Can you work these out from the model? Positions are in its coordinate system, mm. A direction names the side the tool comes from. Round coordinates to 2 decimals unless told otherwise and drop trailing zeros. Order: outer loops, then holes, each group sorted by start corner. A loop starts at its lowest first (then second) coordinate and runs counter-clockwise, first axis right, second up. Notation, with made-up numbers: (33.5, -12) - (48.5, -12) arc R27 cw to (48.5, 16) - close; hole circle Ø10 at (-23, -36). An arc over 180 degrees is marked (long way). Write item = value, one per line.
Autodesk Inventor part; units mm, degrees
ref_plane "Work Plane1" through (0, 0, 10) normal (0, 0, 1) x (1, 0, 0)
ref_plane "YZ Plane" through (0, 0, 0) normal (1, 0, 0) x (0, 1, 0)
ref_plane "XZ Plane" through (0, 0, 0) normal (0, 1, 0) x (-1, 0, 0)
sketch "Sketch1" plane through (0, 0, 0) normal (0, 0, 1) x (1, 0, 0)
  circle A0 centre (0, 0) radius 11.5
extrude "Extrusion1" add sketch "Sketch1" against normal blind 3
sketch "Sketch2" plane through (0, 0, -3) normal (0, 0, -1) x (-1, 0, 0)
  line L0 (-9.8107, 6) -> (-6.8107, 6)
  line L1 (-6.8107, 6) -> (-6.8107, -6)
  line L2 (-6.8107, -6) -> (-9.8107, -6)
  line L3 (-9.8107, -6) -> (-9.8107, 6)
  line L4 (6.8107, 6) -> (9.8107, 6)
  line L5 (9.8107, 6) -> (9.8107, -6)
  line L6 (9.8107, -6) -> (6.8107, -6)
  line L7 (6.8107, -6) -> (6.8107, 6)
  circle A0 centre (0, 0) radius 11.5 construction
  line L8 (0, 11.5) -> (0, -11.5) construction
  arc A1 (-9.8107, 6) -> (-9.8107, -6) centre (0, 0) ccw
  arc A2 (9.8107, -6) -> (9.8107, 6) centre (0, 0) ccw
  arc A3 (9.8107, 6) -> (-9.8107, 6) centre (0, -6.6392) ccw
  arc A4 (-9.8107, -6) -> (9.8107, -6) centre (0, 6.6392) ccw
  circle A5 centre (0, 0) radius 11.5
  point P0 (6.8107, 0)
  dimension "d18" = 3
  dimension "d19" = 12
  dimension "d29" = 16
extrude "Extrusion4" add sketch "Sketch2" along normal blind 18 contours L0 L1 L2 L3 | L5 L6 L7 L4
fillet "Fillet3" radius 6 4 edges at (8.3107, 6, -21) (8.3107, -6, -21) (-8.3107, 6, -21) (-8.3107, -6, -21)
sketch "Sketch3" plane through (9.8107, -6, -3) normal (1, 0, 0) x (0, 0, -1)
  arc A0 (12, 0) -> (12, 12) centre (12, 6) ccw construction
  circle A1 centre (12, 6) radius 4
  point P0 (-3, 6)
  dimension "d23" = 8
extrude "Extrusion5" cut sketch "Sketch3" against normal through all
extrude "Extrusion6" cut sketch "Sketch2" against normal blind 10 contours L3 A1 | A5 A3 | A4 A5 | A2 L5
sketch "Sketch5" plane through (0, 0, 0) normal (0, 0, 1) x (1, 0, 0)
  circle A0 centre (0, 0) radius 8
  dimension "d35" = 16
ref_plane "Work Plane1" through (0, 0, 10) normal (0, 0, 1) x (1, 0, 0)
sketch "Sketch6" plane through (0, 0, 10) normal (0, 0, 1) x (1, 0, 0)
  circle A0 centre (0, 0) radius 8 construction
  circle A1 centre (0, 0) radius 5
  dimension "d37" = 10
loft "Loft1" add profiles "Sketch5", "Sketch6"
sketch "Sketch7" plane through (0, 0, 10) normal (0, 0, 1) x (1, 0, 0)
  circle A0 centre (0, 0) radius 5
  circle A1 centre (0, 0) radius 5 construction
extrude "Extrusion8" add sketch "Sketch7" along normal blind 70
properties part number "wheel hub"
(1) If we section it at C-C (y = 1.5): State how many separate pieces and enclosed holes the cut face has, plus the area to 3 significant figures.
Computed:
separate_pieces = 3
enclosed_holes = 0
area = 915 mm^2
(2) Will these pins go through, and if not, where does the flat tip stop? P1, Ø7, axis at y = 0, z = -15, coming from the -X side; P2, Ø1.5, axis at x = 8.5, z = -7, coming from the -Y side; P3, Ø5, axis at x = 3, z = 9, coming from the -Y side; P4, Ø8, axis at y = 6.5, z = 58, coming from the +X side.
Computed:
P1 = through
P2 = -6
P3 = -5.71
P4 = 4.33
(3) If we section it at A-A (z = -6.5): Write out the boundary of the cut face in (x, y).
Computed:
outline = (-9.81, -6) - (-6.81, -6) - (-6.81, 6) - (-9.81, 6) - close; (6.81, -6) - (9.81, -6) - (9.81, 6) - (6.81, 6) - close
(4) Thinking about a two-plate mould opening in X: for faces 6 (the face through (5.584, -1.758, 7.152)), 7 (the face through (6.811, 0, -10)), 8 (the face through (0, 0, -3)), 9 (the face through (8, 0, -11)), which applies, +X half, -X half, draft (parallel to the pull), parting line (faces both ways), or undercut?
Computed:
face_6 = parting line
face_7 = undercut
face_8 = undercut
face_9 = draft
(5) If we section it at B-B (x = 0): Write out the boundary of the cut face in (y, z), plus the area to 3 significant figures.
Computed:
outline = (-9.36, -3) - (9.36, -3) - (9.36, 0) - (8, 0) - (5, 10) - (5, 80) - (-5, 80) - (-5, 10) - (-8, 0) - (-9.36, 0) - close
area = 886 mm^2
(6) If I drill on line 1 (Y direction, x = -7.4, z = -15); line 2 (X direction, y = -2.5, z = -6); line 3 (Y direction, x = 8.75, z = -10), over which ranges is the centre line in solid material (lowest first)? Write a range as from..to.
Computed:
line_1 = -6..-4, 4..6
line_2 = -9.81..-6.81, 6.81..9.81
line_3 = -6..6
(7) On a 3-axis mill with a long thin cutter (end or side, diameter ignored), from which of +Z, -Z, +X, -X, +Y, -Y can I reach the whole of each face in a straight line? I mean faces 1 (the face through (-1.08, 4.88, 44.51)), 2 (the face through (-9.811, 0, -8)), 3 (the face through (-6.811, 0, -10)), 4 (the face through (8, -6, -9)), 5 (the face through (8, 6, -9)). Say none if no direction works.
Computed:
face_1 = +Z
face_2 = +Z, -Z, -X, +Y, -Y
face_3 = -Z, +Y, -Y
face_4 = -Z, +X, -X, -Y
face_5 = -Z, +X, -X, +Y
(8) If we section it at D-D (z = 61.5): Write out the boundary of the cut face in (x, y).
Computed:
outline = circle Ø10 at (0, 0)
